from build123d import *

# Parameters (mm, degrees)
SKETCH1_W                = 270
SKETCH1_H                = 170
BOSS_EXTRUDE1_DEPTH      = 150
SKETCH2_R                = 12.5
CUT_EXTRUDE1_DEPTH       = 200
BOSS_EXTRUDE2_DEPTH      = 20
BOSS_EXTRUDE2_DEPTH_BACK = 190
SKETCH3_R                = 7.5


with BuildPart() as part:
    # Sketch1 → Boss-Extrude1 (new body)
    with BuildSketch(Plane.XY):
        with Locations((135, 85)):
            Rectangle(SKETCH1_W, SKETCH1_H)
    extrude(amount=BOSS_EXTRUDE1_DEPTH)

    # Sketch2 → Cut-Extrude1 (cut)
    with BuildSketch(Plane(origin=(270, 0, 0), x_dir=(0, 0, -1), z_dir=(1, 0, 0))):
        with Locations((-75, 85)):
            Circle(SKETCH2_R)
    extrude(amount=-CUT_EXTRUDE1_DEPTH, mode=Mode.SUBTRACT)

    # Sketch3 → Boss-Extrude2 (add, two sides: drawn at the far end of the back side and taken through both)
    with BuildSketch(Plane.XZ.offset(-BOSS_EXTRUDE2_DEPTH_BACK)):
        with Locations(Location((55, 15, 0), (0, 0, 270))):
            Circle(SKETCH3_R)
        with Locations(Location((205, 15, 0), (0, 0, 270))):
            Circle(SKETCH3_R)
    extrude(amount=BOSS_EXTRUDE2_DEPTH + BOSS_EXTRUDE2_DEPTH_BACK)


solid = part.part
The listing builds one solid part. Answer for the finished solid, in the listing's coordinates (mm). A direction names the side the tool comes from. Give positions to 0.01 mm unless a question says otherwise; leave off trailing zeros. Write each loop counter-clockwise with the first axis right and the second up, starting at its lowest first coordinate (ties: lowest second). Pieces come first, ordered by that corner, then holes. Notation, with made-up numbers: (-9, -34) -> (19, -34) arc R14 cw to (19, -19) -> close; hole circle Ø4 at (31.5, -0.5). An arc over 180 degrees is marked (long way). One line per question, with ' | ' between items. Start each with the question number.
1. For faces 1 (the flat face through (70, 85, 75)), 2 (the cylindrical face through (212.436, 180.14, 15.976)), 3 (the flat face through (55, 190, 15)), 4 (the cylindrical face through (55.33, -9.86, 22.493)), 5 (the flat face through (205, -20, 15)), determine the directions among +Z, -Z, +X, -X, +Y, -Y from which every point of the face is accessible in a straight line to the end or side of a thin tool.
2. For a pull along Y with two mould halves and no side action, classify faces 6 (the flat face through (55, -20, 15)), 7 (the flat face through (205, 190, 15)), 8 (the cylindrical face through (171.4, 97.394, 76.627)) as pulls with the +Y half, pulls with the -Y half, needs draft (parallel to the pull), parting line crosses it, or undercut.
3. Given pin 1 Ø1.5 at (x, z) = (125, 44.5) entering from -Y; pin 2 Ø22.5 at (y, z) = (85, 75) entering from +X; pin 3 Ø8 at (x, z) = (38, 98) entering from +Y; pin 4 Ø2 at (y, z) = (160, 43.5) entering from -X, each flat-ended and moving along its own axis, determine where each tip first touches the part or whether it passes through.
4. Find the intervals of material crossed by probe 1 along Y at (x, z) = (140.5, 75); probe 2 along Y at (x, z) = (44.5, 118); probe 3 along Y at (x, z) = (189.5, 86.5), in increasing order.
5. Section B-B (z = 15) is taken. Determine the outline of the cut face in (x, y), plus the area to 3 significant figures.
6. Section C-C (y = 85) is taken. Determine the outline of the cut face in (x, z), plus the area to 3 significant figures.
7. Section A-A (x = 205) is taken. Determine the outline of the cut face in (y, z).
8. Section D-D (z = 75) is taken. Determine the outline of the cut face in (x, y).
Response values:
1) face 1: +X | face 2: +Y | face 3: +Z, -Z, +X, -X, +Y | face 4: -Y | face 5: +Z, -Z, +X, -X, -Y
2) face 6: pulls with the -Y half | face 7: pulls with the +Y half | face 8: undercut
3) pin 1: y = 0 | pin 2: x = 70 | pin 3: y = 170 | pin 4: x = 0
4) probe 1: 0 to 72.5, 97.5 to 170 | probe 2: 0 to 170 | probe 3: 0 to 80.1, 89.9 to 170
5) outline: (0, 0) -> (47.5, 0) -> (47.5, -20) -> (62.5, -20) -> (62.5, 0) -> (197.5, 0) -> (197.5, -20) -> (212.5, -20) -> (212.5, 0) -> (270, 0) -> (270, 170) -> (212.5, 170) -> (212.5, 190) -> (197.5, 190) -> (197.5, 170) -> (62.5, 170) -> (62.5, 190) -> (47.5, 190) -> (47.5, 170) -> (0, 170) -> close | area: 47,100 mm2
6) outline: (0, 0) -> (270, 0) -> (270, 62.5) -> (70, 62.5) -> (70, 87.5) -> (270, 87.5) -> (270, 150) -> (0, 150) -> close | area: 35,500 mm2
7) outline: (-20, 7.5) -> (0, 7.5) -> (0, 0) -> (170, 0) -> (170, 7.5) -> (190, 7.5) -> (190, 22.5) -> (170, 22.5) -> (170, 150) -> (0, 150) -> (0, 22.5) -> (-20, 22.5) -> close; hole circle Ø25 at (85, 75)
8) outline: (0, 0) -> (270, 0) -> (270, 72.5) -> (70, 72.5) -> (70, 97.5) -> (270, 97.5) -> (270, 170) -> (0, 170) -> close
